from build123d import *

# Parameters (mm, degrees)
SKETCH2_R           = 2.5
BOSS_EXTRUDE1_DEPTH = 50
CHAMFER1_SIZE       = 0.5
CUT_EXTRUDE1_DEPTH  = 2.3
SKETCH8_R           = 1.782050808
CUT_EXTRUDE2_DEPTH  = 1
CUT_EXTRUDE2_TAPER  = 45


with BuildPart() as part:
    # Sketch2 → Boss-Extrude1 (new body)
    with BuildSketch(Plane(origin=(0, 0, 0), x_dir=(0, 0, -1), z_dir=(1, 0, 0))):
        Circle(SKETCH2_R)
    extrude(amount=-BOSS_EXTRUDE1_DEPTH)

    # Chamfer1
    chamfer1_edges = [part.edges().sort_by_distance(p)[0] for p in [
        (0, 0, 2.5),
    ]]
    chamfer(chamfer1_edges, length=CHAMFER1_SIZE)

    # Sketch6 → Revolve1 (revolve)
    with BuildSketch(Plane.XY):
        with BuildLine():
            Line((-51.5, 0), (-51.5, 4.161437828))
            ThreePointArc((-51.5, 4.161437828), (-50.75, 4.5), (-50, 4.161437828))
            Line((-50, 4.161437828), (-50, 0))
            Line((-50, 0), (-51.5, 0))
        make_face()
    revolve(axis=Axis((-50, 0, 0), (1, 0, 0)))

    # Sketch7 → Cut-Extrude1 (cut)
    with BuildSketch(Plane.ZY.offset(51.5)):
        Polygon((0, 1.732050808), (-1.5, 0.866025404), (-1.5, -0.866025404), (0, -1.732050808), (1.5, -0.866025404), (1.5, 0.866025404), align=None)
    extrude(amount=-CUT_EXTRUDE1_DEPTH, mode=Mode.SUBTRACT)

    # Sketch8 → Cut-Extrude2 (cut)
    with BuildSketch(Plane.ZY.offset(51.5)):
        Circle(SKETCH8_R)
    extrude(amount=-CUT_EXTRUDE2_DEPTH, taper=CUT_EXTRUDE2_TAPER, mode=Mode.SUBTRACT)


solid = part.part
Read the model definition and answer for the solid it produces. Units are mm, in the model's axes. A direction names the side the tool comes from. Coordinates: 2 decimals unless noted, no trailing zeros. Order: outer loops, then holes, each group sorted by start corner. A loop starts at its lowest first (then second) coordinate and runs counter-clockwise, first axis right, second up. Notation, with made-up numbers: (1.5, 4.25) -> (41.5, 4.25) arc R15 ccw to (41.5, 10.25) -> close; hole circle Ø3 at (-2, 38). An arc over 180 degrees is marked (long way). Answer as a JSON object with one key per item and string values.
1) A tool of negligible diameter and unlimited length cuts with its end or side. For faces 4 (the face through (0, 0, 0)), 5 (the face through (-50.341, 1.293, 0.76)), from which of +Z, -Z, +X, -X, +Y, -Y can it reach the whole face along a straight path? Write none if from no direction.
Model answer:
{"face 4": "+Z, -Z, +X, +Y, -Y", "face 5": "-X"}
2) A cutting plane is placed at A-A, the plane x = -18. Determine the outline of the cut face in (y, z).
Model answer:
{"outline": "circle Ø5 at (0, 0)"}
3) Consider line 1 along Z through (x, y) = (-44.5, 1.5); line 2 along X through (y, z) = (1.75, 2.5); line 3 along Z through (x, y) = (-38, -2). Determine where each line is inside the solid, lowest interval first. Write a range as from..to.
Model answer:
{"line 1": "z = -2..2", "line 2": "x = -51.5..-50", "line 3": "z = -1.5..1.5"}
4) Each of these flat-tipped pins is pushed along its axis until it touches: pin 1 (3.5 mm diameter, centred on y = 0.5, z = -0.5, fed in from -X); pin 2 (0.9 mm diameter, centred on x = -50, y = -0.5, fed in from -Z); pin 3 (5 mm diameter, centred on x = -41.5, y = -1.5, fed in from +Z); pin 4 (3 mm diameter, centred on y = -2.5, z = 3.5, fed in from +X). Where does it stop, or does it pass through?
Model answer:
{"pin 1": "stops at x = -51.5", "pin 2": "stops at z = -4.43", "pin 3": "stops at z = 2.5", "pin 4": "stops at x = -50"}
5) The mould has two halves that part along Y. Classify faces 1 (the face through (-50, 0, 1.5)), 2 (the face through (-50, 2, -2)), 3 (the face through (-24.9, -2.44, 0.54)): released by +Y, released by -Y, zero draft, split by the parting line, or undercut.
Model answer:
{"face 1": "undercut", "face 2": "zero draft", "face 3": "split by the parting line"}
